```python
from build123d import *

# Parameters (mm, degrees)
ESQUISSE1_W             = 90
ESQUISSE1_H             = 80
ESQUISSE1_R             = 2.75
ESQUISSE1_R_2           = 3.25
BOSS_EXTRU_1_DEPTH      = 10
ESQUISSE2_R             = 6
ENL_V_MAT_EXTRU_1_DEPTH = 5
ESQUISSE4_R             = 7
ENL_V_MAT_EXTRU_2_DEPTH = 7


with BuildPart() as part:
    # Esquisse1 → Boss.-Extru.1 (new body)
    with BuildSketch(Plane.XY):
        with Locations((-2.432799292, 6.788403994)):
            Rectangle(ESQUISSE1_W, ESQUISSE1_H)
        with Locations((-32.432799292, 36.788403994)):
            Circle(ESQUISSE1_R, mode=Mode.SUBTRACT)
        with Locations((27.567200708, 36.788403994)):
            Circle(ESQUISSE1_R, mode=Mode.SUBTRACT)
        with Locations((27.567200708, -23.211596006)):
            Circle(ESQUISSE1_R, mode=Mode.SUBTRACT)
        with Locations((-32.432799292, -23.211596006)):
            Circle(ESQUISSE1_R, mode=Mode.SUBTRACT)
        with Locations((-37.432799292, 16.788403994)):
            Circle(ESQUISSE1_R_2, mode=Mode.SUBTRACT)
        with Locations((-37.432799292, -3.211596006)):
            Circle(ESQUISSE1_R_2, mode=Mode.SUBTRACT)
        with Locations((32.567200708, 16.788403994)):
            Circle(ESQUISSE1_R_2, mode=Mode.SUBTRACT)
        with Locations((32.567200708, -3.211596006)):
            Circle(ESQUISSE1_R_2, mode=Mode.SUBTRACT)
    extrude(amount=BOSS_EXTRU_1_DEPTH)

    # Esquisse2 → Enlèv. mat.-Extru.1 (cut)
    with BuildSketch(Plane.XY.offset(10)):
        with Locations((-32.432799292, 36.788403994)):
            Circle(ESQUISSE2_R)
        with Locations((27.567200708, 36.788403994)):
            Circle(ESQUISSE2_R)
        with Locations((27.567200708, -23.211596006)):
            Circle(ESQUISSE2_R)
        with Locations((-32.432799292, -23.211596006)):
            Circle(ESQUISSE2_R)
    extrude(amount=-ENL_V_MAT_EXTRU_1_DEPTH, mode=Mode.SUBTRACT)

    # Esquisse4 → Enlèv. mat.-Extru.2 (cut)
    with BuildSketch(Plane(origin=(0, 0, 0), x_dir=(-1, 0, 0), z_dir=(0, 0, -1))):
        with Locations((-32.567200708, 16.788403994)):
            Circle(ESQUISSE4_R)
        with Locations((37.432799292, 16.788403994)):
            Circle(ESQUISSE4_R)
        with Locations((37.432799292, -3.211596006)):
            Circle(ESQUISSE4_R)
        with Locations((-32.567200708, -3.211596006)):
            Circle(ESQUISSE4_R)
    extrude(amount=-ENL_V_MAT_EXTRU_2_DEPTH, mode=Mode.SUBTRACT)


solid = part.part
```
CAD build for the part. Positions are in the model's coordinates, mm. A direction names the side the tool comes from. Round coordinates to 2 decimals unless told otherwise and drop trailing zeros. Order: outer loops, then holes, each group sorted by start corner. A loop starts at its lowest first (then second) coordinate and runs counter-clockwise, first axis right, second up. Notation, with made-up numbers: (14.5, 72) - (48.5, 72) arc R21 cw to (48.5, 108) - close; hole circle Ø8 at (20, 30). An arc over 180 degrees is marked (long way). Answer as CSV lines item,"result". Start each with the question number.
1. Pull direction X, two halves, no side cores. Call faces 1 (the face through (42.567, 6, 5)), 2 (the face through (-35.8, -6.2, 7)), 3 (the face through (-47.433, 6, 5)): +X half, -X half, draft (parallel to the pull), parting line (faces both ways), or undercut.
2. Saw through at A-A, the plane x = -36.5. Write the cut outline in (y, z), and give its area (3 significant figures).
3. Saw through at D-D, the plane y = -8. Write the cut outline in (x, z).
4. Saw through at B-B, the plane y = 38.5. Write the cut outline in (x, z), and give its area (3 significant figures).
5. Drill centre lines: L1, parallel to X at y = 37, z = 3.25; L2, parallel to X at y = -23, z = 7.25; L3, parallel to Y at x = 26.5, z = 7.75. Where is each one in solid material? Low to high. Write a range as [from, to].
6. Tool access for faces 4 (the face through (-35.915, 9.955, 3.451)), 5 (the face through (-31, 34, 5)), 6 (the face through (-3, -33.212, 5)): list every direction of +Z, -Z, +X, -X, +Y, -Y with a clear straight run to the whole face (end or side of a thin tool).
7. Pin check, flat tips, straight feed: pin 1 (8.5 mm diameter, centred on x = -37.43, y = 16.79, fed in from -Z); pin 2 (3.5 mm diameter, centred on x = 30.5, y = -22, fed in from +Z). Stop position of each tip, or through.
8. Saw through at C-C, the plane z = 2. Count the separate pieces of the cut face and the enclosed holes in it, and give its area (3 significant figures).
Model answer:
1,face 1,"+X half"
1,face 2,"undercut"
1,face 3,"-X half"
2,outline,"(-33.21, 0) - (-10.15, 0) - (-10.15, 7) - (-6.32, 7) - (-6.32, 10) - (-18.8, 10) - (-18.8, 5) - (-27.62, 5) - (-27.62, 10) - (-33.21, 10) - close; (-0.1, 7) - (3.73, 7) - (3.73, 0) - (9.85, 0) - (9.85, 7) - (13.68, 7) - (13.68, 10) - (-0.1, 10) - close; (19.9, 7) - (23.73, 7) - (23.73, 0) - (46.79, 0) - (46.79, 10) - (41.2, 10) - (41.2, 5) - (32.38, 5) - (32.38, 10) - (19.9, 10) - close"
2,area,"480 mm²"
3,outline,"(-47.43, 0) - (-42.54, 0) - (-42.54, 7) - (-32.33, 7) - (-32.33, 0) - (27.46, 0) - (27.46, 7) - (37.67, 7) - (37.67, 0) - (42.57, 0) - (42.57, 10) - (-47.43, 10) - close"
4,outline,"(-47.43, 0) - (-34.59, 0) - (-34.59, 5) - (-38.18, 5) - (-38.18, 10) - (-47.43, 10) - close; (-30.28, 0) - (25.41, 0) - (25.41, 5) - (21.82, 5) - (21.82, 10) - (-26.68, 10) - (-26.68, 5) - (-30.28, 5) - close; (29.72, 0) - (42.57, 0) - (42.57, 10) - (33.32, 10) - (33.32, 5) - (29.72, 5) - close"
4,area,"742 mm²"
5,L1,"x = [-47.43, -35.17], [-29.69, 24.83], [30.31, 42.57]"
5,L2,"x = [-47.43, -38.43], [-26.44, 21.57], [33.56, 42.57]"
5,L3,"y = [-33.21, -29.12], [-17.31, 30.88], [42.69, 46.79]"
6,face 4,"-Z"
6,face 5,"+Z"
6,face 6,"+Z, -Z, +X, -X, -Y"
7,pin 1,"stops at z = 7"
7,pin 2,"stops at z = 5"
8,separate pieces,"1"
8,enclosed holes,"8"
8,area,"6,490 mm²"
